```python
from build123d import *

# Parameters (mm, degrees)
F0_R     = 3
F0_W     = 10
F0_H     = 30
F1_DEPTH = 0.6
F2_R     = 2.5
F3_DEPTH = 0.601


with BuildPart() as f1:
    # F0 (on Top) → F1 (new body)
    with BuildSketch(Plane.XY):
        Polygon((0, 80), (0, 0), (80, 0), (80, 80), (70, 80), (10, 80), align=None)
        with Locations((6.5, 6.5)):
            Circle(F0_R, mode=Mode.SUBTRACT)
        with Locations((73.5, 6.5)):
            Circle(F0_R, mode=Mode.SUBTRACT)
        with Locations((6.5, 73.5)):
            Circle(F0_R, mode=Mode.SUBTRACT)
        with Locations((73.5, 73.5)):
            Circle(F0_R, mode=Mode.SUBTRACT)
        with Locations((5, 95)):
            Rectangle(F0_W, F0_H)
        with Locations((75, 95)):
            Rectangle(F0_W, F0_H)
    extrude(amount=F1_DEPTH)

    # F2 (on face) → F3 (cut, through all)
    with BuildSketch(Plane.XY.offset(0.6)):
        with Locations((16.5, 60.5)):
            Circle(F2_R)
        with Locations((63.5, 60.5)):
            Circle(F2_R)
        with Locations((63.5, 19.5)):
            Circle(F2_R)
        with Locations((16.5, 19.5)):
            Circle(F2_R)
    extrude(amount=-F3_DEPTH, mode=Mode.SUBTRACT)


solid = f1.part
```
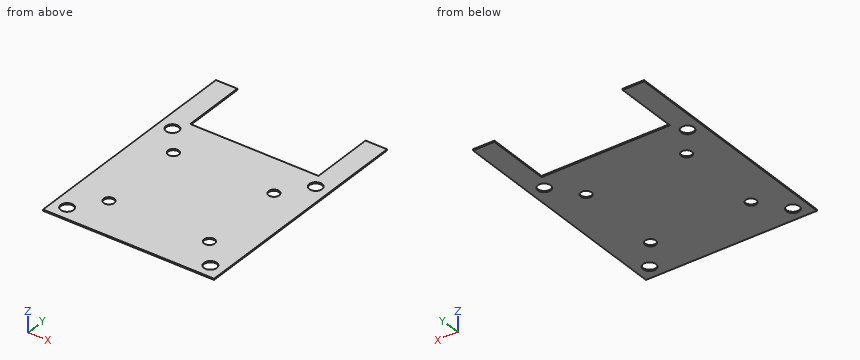
CAD build for the part. Positions are in the model's coordinates, mm. Coordinates: 2 decimals unless noted, no trailing zeros. Write each loop counter-clockwise with the first axis right and the second up, starting at its lowest first coordinate (ties: lowest second). Pieces come first, ordered by that corner, then holes. Notation, with made-up numbers: (11.5, 32.5) -> (33.5, 32.5) arc R21 cw to (33.5, 65.5) -> close; hole circle Ø8 at (3, 73). An arc over 180 degrees is marked (long way). Return JSON: item names as keys, results as strings. Group by question number.
Q1. Cut at A-A, the plane y = 73.5. Give the cut face in (x, z), then the cut area to 3 significant figures.
Q2. Cut at B-B, the plane x = 73.5. Give the cut face in (y, z).
Q3. Flat gauge pins, fed straight in: pin 1 (6.5 mm diameter, centred on x = 16.5, y = 19.5, fed in from -Z); pin 2 (3 mm diameter, centred on x = 16.5, y = 60.5, fed in from -Z). Where does each tip first touch, or does it go through?
Q4. Cut at D-D, the plane y = 91. Give the cut face in (x, z).
Q5. Drill centre lines: line 1 (Y direction, x = 16.5, z = 0.3); line 2 (Y direction, x = 73.5, z = 0.4); line 3 (X direction, y = 92.5, z = 0.35). Where is each one in solid material? Low to high.
Q6. Cut at C-C, the plane z = 0.45. State how many separate pieces and enclosed holes the cut face has, then the cut area to 3 significant figures.
Returned:
{
 "1": {"outline": "(0, 0) -> (3.5, 0) -> (3.5, 0.6) -> (0, 0.6) -> close; (9.5, 0) -> (70.5, 0) -> (70.5, 0.6) -> (9.5, 0.6) -> close; (76.5, 0) -> (80, 0) -> (80, 0.6) -> (76.5, 0.6) -> close", "area": "40.8 mm2"},
 "2": {"outline": "(0, 0) -> (3.5, 0) -> (3.5, 0.6) -> (0, 0.6) -> close; (9.5, 0) -> (70.5, 0) -> (70.5, 0.6) -> (9.5, 0.6) -> close; (76.5, 0) -> (110, 0) -> (110, 0.6) -> (76.5, 0.6) -> close"},
 "3": {"pin 1": "stops at z = 0", "pin 2": "passes through"},
 "4": {"outline": "(0, 0) -> (10, 0) -> (10, 0.6) -> (0, 0.6) -> close; (70, 0) -> (80, 0) -> (80, 0.6) -> (70, 0.6) -> close"},
 "5": {"line 1": "y = 0 to 17, 22 to 58, 63 to 80", "line 2": "y = 0 to 3.5, 9.5 to 70.5, 76.5 to 110", "line 3": "x = 0 to 10, 70 to 80"},
 "6": {"separate pieces": "1", "enclosed holes": "8", "area": "6,810 mm2"}
}
